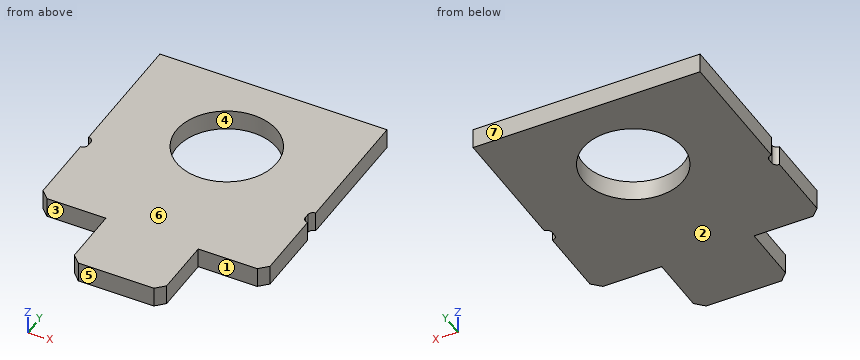
Autodesk Inventor part; units mm, degrees
ref_plane "YZ Plane" through (0, 0, 0) normal (1, 0, 0) x (0, 1, 0)
ref_plane "XZ Plane" through (0, 0, 0) normal (0, 1, 0) x (-1, 0, 0)
ref_plane "XY Plane" through (0, 0, 0) normal (0, 0, 1) x (1, 0, 0)
ref_plane "Work Plane1" through (0, 0, 0) normal (0, 0, 1) x (1, 0, 0)
sketch "Sketch1" plane through (0, 0, 0) normal (0, 0, 1) x (1, 0, 0)
  circle A0 centre (-67.9848, -106.1458) radius 30
  line L0 (0, -139.7083) -> (0, -24)
  line L1 (-95.6323, -230.1458) -> (-40.3675, -230.1458)
  line L2 (-40.3675, -230.1458) -> (-40.3675, -106.1458)
  line L3 (-40.3675, -106.1458) -> (-95.6323, -106.1458)
  line L4 (-95.6323, -106.1458) -> (-95.6323, -230.1458)
  line L5 (-135.9998, -189.7783) -> (0, -189.7783)
  line L6 (0, -189.7783) -> (0, -53.7785)
  line L7 (0, -53.7785) -> (-135.9998, -53.7785)
  line L8 (-135.9998, -53.7785) -> (-135.9998, -189.7783)
  line L9 (-147.9998, -163.7083) -> (-135.9998, -163.7083)
  line L10 (-135.9998, -189.7783) -> (-135.9998, -163.7083)
  line L11 (-135.9998, -189.7783) -> (-147.9998, -189.7783)
  line L12 (-147.9998, -189.7783) -> (-147.9998, -163.7083)
  point P0 (0, 0)
  point P1 (-40.3675, -230.1458)
  point P2 (0, -189.7783)
  point P3 (-40.3675, -189.7783)
  point P4 (-95.6323, -189.7783)
extrude "Extrusion1" add sketch "Sketch1" along normal blind 12 contours A0 L4 L5 L8 L7 L0 L6 L2 | A0 L2 L5 L4 | L5 L2 L1 L4
chamfer "Chamfer1" distance 5 angle 45 4 edges at (-135.9998, -189.7783, 6) (-95.6323, -230.1458, 6) (-40.3675, -230.1458, 6) (0, -189.7783, 6)
sketch "Sketch4" plane through (0, 0, 0) normal (0, 0, -1) x (-1, 0, 0)
  line L0 (135.9998, -163.7083) -> (135.9998, -139.7083)
  line L1 (135.9998, -136.7194) -> (135.9998, 252.4278)
  line L2 (135.9998, -136.7194) -> (135.9998, -139.7083) construction
  line L3 (135.9998, -53.7785) -> (135.9998, -184.7783)
  line L4 (132.9998, -136.7194) -> (132.9998, -139.7083)
  line L5 (138.9998, -139.7083) -> (138.9998, -136.7194)
  arc A0 (138.9998, -136.7194) -> (132.9998, -136.7194) centre (135.9998, -136.7194) ccw
  arc A1 (132.9998, -139.7083) -> (138.9998, -139.7083) centre (135.9998, -139.7083) ccw
  point P0 (0, 0)
  point P1 (135.9998, -138.2139)
  point P2 (135.9998, -142.7083)
  point P3 (135.9998, -133.7194)
  dimension "d6" = 6
extrude "Extrusion2" cut sketch "Sketch4" against normal through all contours A1 L4 A0 L1 L3 L0
ref_plane "Work Plane2" through (-147.9998, 57.8542, 0) normal (-1, 0, 0) x (0, -1, 0)
ref_plane "Work Plane3" through (-67.9999, -53.7785, 12) normal (1, 0, 0) x (0, 0, -1)
mirror "Mirror1" about plane through (-67.9999, -53.7785, 12) normal (1, 0, 0) of "Extrusion2"
sketch "Sketch7" plane through (0, 0, 12) normal (0, 0, 1) x (1, 0, 0)
  circle A0 centre (-67.9848, -106.1458) radius 30
  arc A1 (-3, -139.7083) -> (0, -142.7083) centre (0, -139.7083) ccw
  line L0 (-3, -139.7083) -> (-3, -136.7194)
  arc A2 (0, -133.7194) -> (-3, -136.7194) centre (0, -136.7194) ccw
  line L1 (0, -133.7194) -> (0, -53.7785)
  line L2 (0, -53.7785) -> (-135.9998, -53.7785)
  line L3 (-135.9998, -53.7785) -> (-135.9998, -133.7194)
  arc A3 (-132.9998, -136.7194) -> (-135.9998, -133.7194) centre (-135.9998, -136.7194) ccw
  line L4 (-132.9998, -136.7194) -> (-132.9998, -139.7083)
  arc A4 (-135.9998, -142.7083) -> (-132.9998, -139.7083) centre (-135.9998, -139.7083) ccw
  line L5 (-135.9998, -142.7083) -> (-135.9998, -184.7783)
  line L6 (-130.9998, -189.7783) -> (-135.9998, -184.7783)
  line L7 (-130.9998, -189.7783) -> (-95.6323, -189.7783)
  line L8 (-95.6323, -189.7783) -> (-95.6323, -225.1458)
  line L9 (-90.6323, -230.1458) -> (-95.6323, -225.1458)
  line L10 (-90.6323, -230.1458) -> (-45.3675, -230.1458)
  line L11 (-40.3675, -225.1458) -> (-45.3675, -230.1458)
  line L12 (-40.3675, -225.1458) -> (-40.3675, -189.7783)
  line L13 (-40.3675, -189.7783) -> (-5, -189.7783)
  line L14 (0, -184.7783) -> (-5, -189.7783)
  line L15 (0, -184.7783) -> (0, -142.7083)
  point P0 (0, 0)
properties part number "internal"
Could you check a few things on this model? Use its own coordinates, in mm. Face numbers are marked on the shaded views. A direction names the side the tool comes from. Round coordinates to 2 decimals unless told otherwise and drop trailing zeros. Write each loop counter-clockwise with the first axis right and the second up, starting at its lowest first coordinate (ties: lowest second). Pieces come first, ordered by that corner, then holes.
(1) If I drill on probe 1 along X at (y, z) = (-217.5, 5.5); probe 2 along Y at (x, z) = (-23.5, 1.5); probe 3 along X at (y, z) = (-138, 6.25), over which ranges is the centre line in solid material (lowest first)?
Findings below:
probe 1: x = -95.63 to -40.37
probe 2: y = -189.78 to -53.78
probe 3: x = -133 to -3
(2) For pin 1 (6 mm diameter, centred on x = -110, z = 3, fed in from -Y); pin 2 (3.5 mm diameter, centred on y = -214.5, z = 3.5, fed in from +X); pin 3 (3.5 mm diameter, centred on y = -138, z = 7.5, fed in from +X), each with a flat end and sliding along its axis, tell me the tip position at first contact or that it passes through.
Findings below:
pin 1: stops at y = -189.78
pin 2: stops at x = -40.37
pin 3: stops at x = -2.96
(3) Suppose I cut it at D-D on y = -192. Write out the boundary of the cut face in (x, z).
Findings below:
outline: (-95.63, 0) - (-40.37, 0) - (-40.37, 12) - (-95.63, 12) - close
(4) Suppose I cut it at A-A on y = -118. Write out the boundary of the cut face in (x, z), and give its area (3 significant figures).
Findings below:
outline: (-136, 0) - (-95.54, 0) - (-95.54, 12) - (-136, 12) - close; (-40.43, 0) - (0, 0) - (0, 12) - (-40.43, 12) - close
area: 971 mm2
(5) Suppose I cut it at C-C on z = 10. Write out the boundary of the cut face in (x, y).
Findings below:
outline: (-136, -184.78) - (-131, -189.78) - (-95.63, -189.78) - (-95.63, -225.15) - (-90.63, -230.15) - (-45.37, -230.15) - (-40.37, -225.15) - (-40.37, -189.78) - (-5, -189.78) - (0, -184.78) - (0, -142.71) arc R3 cw to (-3, -139.71) - (-3, -136.72) arc R3 cw to (0, -133.72) - (0, -53.78) - (-136, -53.78) - (-136, -133.72) arc R3 cw to (-133, -136.72) - (-133, -139.71) arc R3 cw to (-136, -142.71) - close; hole circle Ø60 at (-67.98, -106.15)
(6) Suppose I cut it at B-B on x = -65. Write out the boundary of the cut face in (y, z), and give its area (3 significant figures).
Findings below:
outline: (-230.15, 0) - (-136, 0) - (-136, 12) - (-230.15, 12) - close; (-76.29, 0) - (-53.78, 0) - (-53.78, 12) - (-76.29, 12) - close
area: 1,400 mm2
(7) Which directions (+Z, -Z, +X, -X, +Y, -Y) give clear straight access to the entire face, cutting with the end or side of a thin tool? Please do the marked faces 1, 2 and 3.
Findings below:
face 1: +Z, -Z, +X, -Y
face 2: -Z, +X, -X, +Y, -Y
face 3: +Z, -Z, -X, -Y
(8) Thinking about a two-plate mould opening in Y: for the marked faces 4, 5, 6 and 7, which applies, +Y half, -Y half, draft (parallel to the pull), parting line (faces both ways), or undercut?
Findings below:
face 4: undercut
face 5: -Y half
face 6: draft
face 7: +Y half
